Read the model definition and answer for the solid it produces. Units are mm, in the model's axes. A direction names the side the tool comes from. Give positions to 0.01 mm unless a question says otherwise; leave off trailing zeros. Order: outer loops, then holes, each group sorted by start corner. A loop starts at its lowest first (then second) coordinate and runs counter-clockwise, first axis right, second up. Notation, with made-up numbers: (-22, 50) -> (-14, 50) arc R22 cw to (-14, 80) -> close; hole circle Ø5 at (41.25, 64). An arc over 180 degrees is marked (long way). Use one line per item in the form item = value.
```python
from build123d import *

# Parameters (mm, degrees)
F0_W      = 250
F0_H      = 185
F1_DEPTH  = 4
F3_DEPTH  = 1.5
F5_DEPTH  = 5
F6_R      = 2
F7_DEPTH  = 25
F8_DEPTH  = 20
F10_DEPTH = 4.001
F12_DEPTH = 5
F13_R     = 5


with BuildPart() as f1:
    # F0 (on Top) → F1 (new body)
    with BuildSketch(Plane.XY):
        with Locations((45.8660066128, 4.6654982038)):
            Rectangle(F0_W, F0_H)
    extrude(amount=F1_DEPTH)

    # F2 (on face) → F3 (cut)
    with BuildSketch(Plane.XY.offset(4)):
        with BuildLine():
            ThreePointArc((53.8660066128, 80.1654982038), (51.5228608623, 85.8223524533), (45.8660066128, 88.1654982038))
            ThreePointArc((45.8660066128, 88.1654982038), (40.2091523633, 85.8223524533), (37.8660066128, 80.1654982038))
            Line((37.8660066128, 80.1654982038), (37.8660066128, -62.8345017962))
            ThreePointArc((37.8660066128, -62.8345017962), (40.2091523633, -68.4913560457), (45.8660066128, -70.8345017962))
            ThreePointArc((45.8660066128, -70.8345017962), (51.5228608623, -68.4913560457), (53.8660066128, -62.8345017962))
            Line((53.8660066128, -62.8345017962), (53.8660066128, 80.1654982038))
        make_face()
    extrude(amount=-F3_DEPTH, mode=Mode.SUBTRACT)

    # F4 (on face) → F5 (cut)
    with BuildSketch(Plane.XY.offset(2.5)):
        with BuildLine():
            Line((48.3660066128, -62.8345017962), (48.3660066128, 80.1654982038))
            ThreePointArc((48.3660066128, 80.1654982038), (45.8660066128, 82.6654982038), (43.3660066128, 80.1654982038))
            Line((43.3660066128, 80.1654982038), (43.3660066128, -62.8345017962))
            ThreePointArc((43.3660066128, -62.8345017962), (45.8660066128, -65.3345017962), (48.3660066128, -62.8345017962))
        make_face()
    extrude(amount=-F5_DEPTH, mode=Mode.SUBTRACT)

    # F6 (on face) → F7 (cut)
    with BuildSketch(Plane.XY.offset(4)):
        with Locations((163.1860066128, 37.1654982038)):
            Circle(F6_R)
        with Locations((163.1860066128, -73.8345017962)):
            Circle(F6_R)
    extrude(amount=-F7_DEPTH, mode=Mode.SUBTRACT)

    # F8 (add): a face of the model
    f8_faces = [f1.faces().sort_by_distance(p)[0] for p in [
        (170.8660066128, 4.6654982038, 2),
    ]]
    extrude(f8_faces, amount=F8_DEPTH)

    # F9 (on face) → F10 (cut, through all)
    with BuildSketch(Plane.XY.offset(4)):
        with BuildLine():
            Line((178.3660066128, 87.1654982038), (178.0660066128, 87.1654982038))
            ThreePointArc((178.0660066128, 87.1654982038), (174.8840260974, 85.8474787192), (173.5660066128, 82.6654982038))
            Line((173.5660066128, 82.6654982038), (173.5660066128, -78.3345017962))
            ThreePointArc((173.5660066128, -78.3345017962), (174.8840260974, -81.5164823115), (178.0660066128, -82.8345017962))
            Line((178.0660066128, -82.8345017962), (178.3660066128, -82.8345017962))
            ThreePointArc((178.3660066128, -82.8345017962), (181.5479871281, -81.5164823115), (182.8660066128, -78.3345017962))
            Line((182.8660066128, -78.3345017962), (182.8660066128, 82.6654982038))
            ThreePointArc((182.8660066128, 82.6654982038), (181.5479871281, 85.8474787192), (178.3660066128, 87.1654982038))
        make_face()
    extrude(amount=-F10_DEPTH, mode=Mode.SUBTRACT)

    # F11 (on face) → F12 (join)
    with BuildSketch(Plane(origin=(0, 0, 0), x_dir=(1, 0, 0), z_dir=(0, 0, -1))):
        with BuildLine():
            Line((190.8660066128, -97.1654982038), (190.8660066128, 87.8345017962))
            Line((190.8660066128, 87.8345017962), (164.8207604885, 87.8345017962))
            Line((164.8207604885, 87.8345017962), (164.8207604885, 74.9867082732))
            ThreePointArc((164.8207604885, 74.9867082732), (165.0925096617, 74.4388577544), (165.1860066128, 73.8345017962))
            ThreePointArc((165.1860066128, 73.8345017962), (165.0925096617, 73.2301458379), (164.8207604885, 72.6822953191))
            Line((164.8207604885, 72.6822953191), (164.8207604885, -36.0132917268))
            ThreePointArc((164.8207604885, -36.0132917268), (165.0925096617, -36.5611422456), (165.1860066128, -37.1654982038))
            ThreePointArc((165.1860066128, -37.1654982038), (165.0925096617, -37.7698541621), (164.8207604885, -38.3177046809))
            Line((164.8207604885, -38.3177046809), (164.8207604885, -97.1654982038))
            Line((164.8207604885, -97.1654982038), (190.8660066128, -97.1654982038))
        make_face()
        with BuildLine():
            ThreePointArc((182.8660066128, -82.6654982038), (181.5479871281, -85.8474787192), (178.3660066128, -87.1654982038))
            Line((178.3660066128, -87.1654982038), (178.0660066128, -87.1654982038))
            ThreePointArc((178.0660066128, -87.1654982038), (174.8840260974, -85.8474787192), (173.5660066128, -82.6654982038))
            Line((173.5660066128, -82.6654982038), (173.5660066128, 78.3345017962))
            ThreePointArc((173.5660066128, 78.3345017962), (174.8840260974, 81.5164823115), (178.0660066128, 82.8345017962))
            Line((178.0660066128, 82.8345017962), (178.3660066128, 82.8345017962))
            ThreePointArc((178.3660066128, 82.8345017962), (181.5479871281, 81.5164823115), (182.8660066128, 78.3345017962))
            Line((182.8660066128, 78.3345017962), (182.8660066128, -82.6654982038))
        make_face(mode=Mode.SUBTRACT)
        with BuildLine():
            Line((178.0660066128, -87.1654982038), (178.3660066128, -87.1654982038))
            ThreePointArc((178.3660066128, -87.1654982038), (181.5479871281, -85.8474787192), (182.8660066128, -82.6654982038))
            Line((182.8660066128, -82.6654982038), (182.8660066128, 78.3345017962))
            ThreePointArc((182.8660066128, 78.3345017962), (181.5479871281, 81.5164823115), (178.3660066128, 82.8345017962))
            Line((178.3660066128, 82.8345017962), (178.0660066128, 82.8345017962))
            ThreePointArc((178.0660066128, 82.8345017962), (174.8840260974, 81.5164823115), (173.5660066128, 78.3345017962))
            Line((173.5660066128, 78.3345017962), (173.5660066128, -82.6654982038))
            ThreePointArc((173.5660066128, -82.6654982038), (174.8840260974, -85.8474787192), (178.0660066128, -87.1654982038))
        make_face()
    extrude(amount=F12_DEPTH)

    # F13
    f13_edges = [f1.edges().sort_by_distance(p)[0] for p in [
        (190.866007, 97.165498, -0.5),
        (-79.133993, 97.165498, 2),
        (-79.133993, -87.834502, 2),
        (190.866007, -87.834502, -0.5),
        (164.82076, -87.834502, -2.5),
        (164.82076, 97.165498, -2.5),
    ]]
    fillet(f13_edges, radius=F13_R)


solid = f1.part
```
Item 1: The part is cut by section C-C on x = 20. Give the vertices of the cut face in (y, z), and give its area (3 significant figures).
Checks:
outline = (-87.83, 0) -> (97.17, 0) -> (97.17, 4) -> (-87.83, 4) -> close
area = 740 mm²
Item 2: Given pin 1 Ø2 at (y, z) = (48.5, -2) entering from -X; pin 2 Ø8 at (x, y) = (44.5, 30.5) entering from +Z, each flat-ended and moving along its own axis, determine where each tip first touches the part or whether it passes through.
Checks:
pin_1 = 164.82
pin_2 = 2.5
Item 3: Determine the mould class of faces 1 (the flat face through (54, 97.165, 3)), 2 (the flat face through (49, 10, 2.5)), 3 (the cylindrical face through (-77.71, -86.33, 2.03)) for opening direction Y: +Y half, -Y half, draft (parallel to the pull), parting line (faces both ways), or undercut.
Checks:
face_1 = +Y half
face_2 = undercut
face_3 = -Y half
Item 4: Which of the six approach directions +Z, -Z, +X, -X, +Y, -Y give full straight-line access (tool end or side, diameter ignored) to faces 4 (the flat face through (178, 1, 0)), 5 (the cylindrical face through (189.44, -86.33, -0.56)), 6 (the flat face through (16, 3, 0)), 7 (the cylindrical face through (166.247, 95.662, -2.535)), 8 (the cylindrical face through (166.247, -86.331, -2.535))?
Checks:
face_4 = +Z
face_5 = +Z, -Z, +X, -Y
face_6 = -Z, -X, +Y, -Y
face_7 = -Z, -X, +Y
face_8 = -Z, -X, -Y
Item 5: The part is cut by section A-A on y = 54.5. Give the vertices of the cut face in (x, z), and give its area (3 significant figures).
Checks:
outline = (-79.13, 0) -> (43.37, 0) -> (43.37, 2.5) -> (37.87, 2.5) -> (37.87, 4) -> (-79.13, 4) -> close; (48.37, 0) -> (164.82, 0) -> (164.82, -5) -> (190.87, -5) -> (190.87, 4) -> (182.87, 4) -> (182.87, 0) -> (173.57, 0) -> (173.57, 4) -> (53.87, 4) -> (53.87, 2.5) -> (48.37, 2.5) -> close
area = 1,140 mm²
Item 6: The part is cut by section B-B on z = -3. Give the vertices of the cut face in (x, y).
Checks:
outline = (164.82, -82.83) arc R5 ccw to (169.82, -87.83) -> (185.87, -87.83) arc R5 ccw to (190.87, -82.83) -> (190.87, 92.17) arc R5 ccw to (185.87, 97.17) -> (169.82, 97.17) arc R5 ccw to (164.82, 92.17) -> (164.82, 38.32) arc R2 cw to (164.82, 36.01) -> (164.82, -72.68) arc R2 cw to (164.82, -74.99) -> close
Item 7: Straight lines are drawn through the part: L1, parallel to X at y = 24, z = 3.5; L2, parallel to Z at x = 97.5, y = -47; L3, parallel to X at y = 20, z = -2.25. For each, find the intervals that lie inside material, in ascending order. Write a range as from..to.
Checks:
L1 = -79.13..37.87, 53.87..173.57, 182.87..190.87
L2 = 0..4
L3 = 164.82..190.87
